```python
from build123d import *

# Parameters (mm, degrees)
BOSS_EXTRUDE1_DEPTH = 2.5


with BuildPart() as part:
    # Model → Boss-Extrude1 (new, symmetric)
    with BuildSketch(Plane.XY):
        with BuildLine():
            ThreePointArc((717.900029607, 115.214424851), (670.427821467, 108.213195948), (650.508452339, 64.557194238))
            ThreePointArc((650.508452339, 64.557194238), (653.283849766, 52.747710067), (660.139069353, 42.739078209))
            ThreePointArc((660.139069353, 42.739078209), (657.792156458, 25.994108012), (641.047186261, 23.647195117))
            ThreePointArc((641.047186261, 23.647195117), (644.900795358, 20.115585583), (649.047156658, 16.932779125))
            ThreePointArc((649.047156658, 16.932779125), (696.519364798, 23.934008028), (716.438733926, 67.590009739))
            ThreePointArc((716.438733926, 67.590009739), (713.663336498, 79.399493909), (706.808116912, 89.408125767))
            ThreePointArc((706.808116912, 89.408125767), (709.155029807, 106.153095964), (725.900000004, 108.500008859))
            ThreePointArc((725.900000004, 108.500008859), (722.046390907, 112.031618393), (717.900029607, 115.214424851))
        make_face()
        with BuildLine():
            Line((697.355906954, 72.047955987), (686.946544773, 80.782447954))
            ThreePointArc((686.946544773, 80.782447954), (686.354148507, 82.410043316), (685.240807709, 81.08321542))
            Line((685.240807709, 81.08321542), (671.532142065, 76.093669174))
            Line((671.532142065, 76.093669174), (668.825234868, 60.742035599))
            Line((668.825234868, 60.742035599), (680.766685935, 50.721968413))
            Line((680.766685935, 50.721968413), (695.415044199, 56.053534802))
            Line((695.415044199, 56.053534802), (697.948303219, 70.420360624))
            ThreePointArc((697.948303219, 70.420360624), (699.061644018, 71.747188521), (697.355906954, 72.047955987))
        make_face(mode=Mode.SUBTRACT)
    extrude(amount=BOSS_EXTRUDE1_DEPTH, both=True)


solid = part.part
```
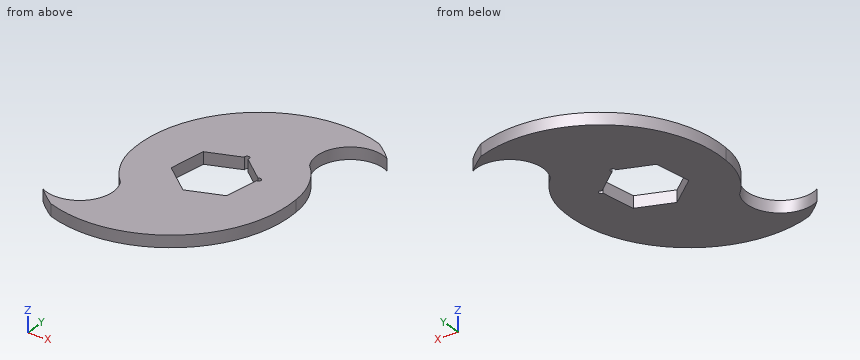
Work out the finished part from the listing and answer in its coordinate system (mm). Give positions to 0.01 mm unless a question says otherwise; leave off trailing zeros. Loops run counter-clockwise (first coordinate to the right, second up) from the corner with the lowest first, then second, coordinate; pieces in that order, holes last. Notation, with made-up numbers: (-23.75, -34) - (-12.75, -34) arc R19 cw to (-12.75, -9) - close; hole circle Ø7 at (12, -18). An arc over 180 degrees is marked (long way). One line per question, with ' | ' between items.
(1) The part is cut by section C-C (y = 74). Write down the section's boundary in (x, z).
Recorded:
outline: (650.74, -2.5) - (671.16, -2.5) - (671.16, 2.5) - (650.74, 2.5) - close; (695.03, -2.5) - (715.51, -2.5) - (715.51, 2.5) - (695.03, 2.5) - close
(2) Each of these flat-tipped pins is pushed along its axis until it touches: pin 1 Ø1.2 at (x, y) = (698.12, 71.41) entering from -Z; pin 2 Ø3 at (y, z) = (39, -1.5) entering from -X; pin 3 Ø1 at (y, z) = (55, 1) entering from -X; pin 4 Ø1.5 at (y, z) = (51.5, 0.5) entering from +X. Where does it stop, or does it pass through?
Recorded:
pin 1: passes through | pin 2: stops at x = 661.14 | pin 3: stops at x = 652.21 | pin 4: stops at x = 715.15
(3) The part is cut by section B-B (z = -1.25). Write down the section's boundary in (x, y), then the cut area to 3 significant figures.
Recorded:
outline: (641.05, 23.65) arc R60 ccw to (649.05, 16.93) arc R50.21 ccw to (716.44, 67.59) arc R33 ccw to (706.81, 89.41) arc R14.04 cw to (725.9, 108.5) arc R60 ccw to (717.9, 115.21) arc R50.21 ccw to (650.51, 64.56) arc R33 ccw to (660.14, 42.74) arc R14.04 cw to start; hole (668.83, 60.74) - (680.77, 50.72) - (695.42, 56.05) - (697.95, 70.42) arc R1 ccw (long way) to (697.36, 72.05) - (686.95, 80.78) arc R1 ccw (long way) to (685.24, 81.08) - (671.53, 76.09) - close | area: 4,680 mm²
(4) The part is cut by section A-A (x = 653). Write down the section's boundary in (y, z), then the cut area to 3 significant figures.
Recorded:
outline: (15.66, -2.5) - (22.85, -2.5) - (22.85, 2.5) - (15.66, 2.5) - close; (53.41, -2.5) - (84.07, -2.5) - (84.07, 2.5) - (53.41, 2.5) - close | area: 189 mm²
(5) The part is cut by section D-D (x = 700.5). Write down the section's boundary in (y, z).
Recorded:
outline: (27.26, -2.5) - (118.29, -2.5) - (118.29, 2.5) - (27.26, 2.5) - close
(6) Straight lines are drawn through the part: probe 1 along Y at (x, z) = (698.5, -1.4); probe 2 along Y at (x, z) = (683.5, -1.85); probe 3 along X at (y, z) = (64, 1.6). For each, find the intervals that lie inside material, in ascending order.
Recorded:
probe 1: y = 25.5 to 70.48, 72.33 to 118.24 | probe 2: y = 16.88 to 51.72, 80.45 to 115.29 | probe 3: x = 650.54 to 669.4, 696.82 to 716.56
